```python
from build123d import *

# Parameters (mm, degrees)
SKETCH1_R           = 3.81
BOSS_EXTRUDE1_DEPTH = 10
CHAMFER1_SIZE       = 0.75
FILLET1_R           = 2.5
CHAMFER2_SIZE       = 0.75


with BuildPart() as part:
    # Sketch1 → Boss-Extrude1 (new body)
    # profile 1 of 2: a face of its own
    with BuildSketch(Plane(origin=(0, 0, 0), x_dir=(1, 0, 0), z_dir=(0, 1, 0))):
        with BuildLine():
            Line((-6.505382387, 22.515382387), (-7.919595949, 23.929595949))
            ThreePointArc((-7.919595949, 23.929595949), (0, 4.81), (7.919595949, 23.929595949))
            Line((7.919595949, 23.929595949), (6.505382387, 22.515382387))
            ThreePointArc((6.505382387, 22.515382387), (0, 6.81), (-6.505382387, 22.515382387))
        make_face()
    # profile 2 of 2: a face of its own
    with BuildSketch(Plane(origin=(0, 0, 0), x_dir=(1, 0, 0), z_dir=(0, 1, 0))):
        with BuildLine():
            ThreePointArc((8.919585019, 9.236448267), (0, 4.81), (-8.919585019, 9.236448267))
            ThreePointArc((-8.919585019, 9.236448267), (-6.608257967, 4.872922521), (-5.81, 0))
            ThreePointArc((-5.81, 0), (0, -5.81), (5.81, 0))
            ThreePointArc((5.81, 0), (6.608257967, 4.872922521), (8.919585019, 9.236448267))
        make_face()
        with Locations(Location((0, 0, 0), (0, 0, 270))):
            Circle(SKETCH1_R, mode=Mode.SUBTRACT)
    extrude(amount=BOSS_EXTRUDE1_DEPTH)

    # Chamfer1
    chamfer1_edges = [part.edges().sort_by_distance(p)[0] for p in [
        (0, 0, -3.81),
        (0, 10, -3.81),
    ]]
    chamfer(chamfer1_edges, length=CHAMFER1_SIZE)

    # Fillet1
    # the kernel refuses this fillet: 2.5 mm, written as the material it takes off along each edge
    with BuildSketch(Plane(origin=(6.505382387, -5, -22.515382387), x_dir=(0.7071067811865479, 0, -0.707106781186547), z_dir=(0, 1, 0))) as fillet1_piece_1:
        with BuildLine():
            CenterArc((2.232142857, -2.489198605), FILLET1_R, 95.327997904, 72.388325655)
            Line((-0.210622711, -1.957318561), (-0.259478022, -1.94668096))
            ThreePointArc((-0.259478022, -1.94668096), (-0.102520236, -0.978959627), (-0.05, 0))
            Line((-0.05, 0), (0, 0.05))
            ThreePointArc((0, 0.05), (1, 0.05), (1.995357143, 0.049783972))
            Line((1.995357143, 0.049783972), (2, 0))
        make_face()
    extrude(amount=20, mode=Mode.SUBTRACT)
    with BuildSketch(Plane(origin=(-6.505382387, -5, -22.515382387), x_dir=(-0.7071067811865465, 0, -0.7071067811865487), z_dir=(0, 1, 0))) as fillet1_piece_2:
        with BuildLine():
            CenterArc((2.232142857, 2.489198605), FILLET1_R, 192.283676441, 72.388325655)
            Line((-0.210622711, 1.957318561), (-0.259478022, 1.94668096))
            ThreePointArc((-0.259478022, 1.94668096), (-0.102520236, 0.978959627), (-0.05, 0))
            Line((-0.05, 0), (0, -0.05))
            ThreePointArc((0, -0.05), (1, -0.05), (1.995357143, -0.049783972))
            Line((1.995357143, -0.049783972), (2, 0))
        make_face()
    extrude(amount=20, mode=Mode.SUBTRACT)

    # Chamfer2
    chamfer2_edges = [part.edges().sort_by_distance(p)[0] for p in [
        (0, 0, -6.81),
        (0, 10, -6.81),
        (-7.348479111, 0, -22.485272721),
        (7.348479111, 0, -22.485272721),
        (-7.348479111, 10, -22.485272721),
        (7.348479111, 10, -22.485272721),
    ]]
    chamfer(chamfer2_edges, length=CHAMFER2_SIZE)


solid = part.part
```
Can you work these out from the model? Positions are in its coordinate system, mm. A direction names the side the tool comes from. Round coordinates to 2 decimals unless told otherwise and drop trailing zeros. Loops run counter-clockwise (first coordinate to the right, second up) from the corner with the lowest first, then second, coordinate; pieces in that order, holes last.
Item 1: Suppose I cut it at C-C, the plane y = 5. Write out the boundary of the cut face in (x, z), then the cut area to 3 significant figures.
Item 2: Will these pins go through, and if not, where does the flat tip stop? pin 1 Ø1 at (x, z) = (5, 2) entering from -Y; pin 2 Ø6 at (y, z) = (8, -20.5) entering from +X; pin 3 Ø10 at (x, z) = (-1.5, -12) entering from -Y; pin 4 Ø2 at (y, z) = (4, -6.5) entering from +X.
Item 3: Suppose I cut it at B-B, the plane x = 0. Write out the boundary of the cut face in (y, z), then the cut area to 3 significant figures.
Item 4: Suppose I cut it at A-A, the plane z = -16.01. Write out the boundary of the cut face in (x, y), then the cut area to 3 significant figures.
Item 5: Which directions (+Z, -Z, +X, -X, +Y, -Y) give clear straight access to the entire face, cutting with the end or side of a thin tool? Please do faces 5 (the cylindrical face through (7.35, 4.94, -22.51)), 6 (the cylindrical face through (-6.63, 4.93, -4.94)).
Item 6: If we mould it in two halves opening along Z, with no side actions, what happens to faces 1 (the cylindrical face through (-7.347, 4.94, -22.463)), 2 (the flat face through (-0.1, 0, -5.6)), 3 (the cylindrical face through (-0.13, 4.93, 5.81)), 4 (the cylindrical face through (11.18, 4.93, -16.66))? For each: +Z half, -Z half, draft (parallel to the pull), parting line (faces both ways), or undercut.
Item 7: Please list where these lines run through material, in increasing order: L1, parallel to X at y = 6.5, z = -16.01; L2, parallel to Z at x = -2, y = 5.5; L3, parallel to X at y = 1, z = -14.
Reported:
1. outline: (-8.92, -9.24) arc R11.2 ccw to (-7.92, -23.93) arc R2.5 ccw to (-7.74, -20.98) arc R9.2 cw (long way) to (7.74, -20.98) arc R2.5 ccw to (7.92, -23.93) arc R11.2 ccw to (8.92, -9.24) arc R15.27 cw to (5.81, 0) arc R5.81 ccw to (-5.81, 0) arc R15.27 cw to start; hole circle Ø7.62 at (0, 0)
1. area: 172 mm2
2. pin 1: stops at y = 0
2. pin 2: stops at x = 11.1
2. pin 3: stops at y = 0.67
2. pin 4: stops at x = 7.78
3. outline: (0, -6.06) - (0.75, -6.81) - (9.25, -6.81) - (10, -6.06) - (10, -4.56) - (9.25, -3.81) - (0.75, -3.81) - (0, -4.56) - close; (0, 4.56) - (0.75, 3.81) - (9.25, 3.81) - (10, 4.56) - (10, 5.81) - (0, 5.81) - close
3. area: 48.3 mm2
4. outline: (-11.2, 0) - (-9.95, 0) - (-9.2, 0.75) - (-9.2, 9.25) - (-9.95, 10) - (-11.2, 10) - close; (9.2, 0.75) - (9.95, 0) - (11.2, 0) - (11.2, 10) - (9.95, 10) - (9.2, 9.25) - close
4. area: 38.9 mm2
5. face 5: +Y, -Y
5. face 6: +Z, -X, +Y, -Y
6. face 1: undercut
6. face 2: draft
6. face 3: +Z half
6. face 4: parting line
7. L1: x = -11.2 to -9.2, 9.2 to 11.2
7. L2: z = -7.03 to -3.24, 3.24 to 5.45
7. L3: x = -11.02 to -8.98, 8.98 to 11.02
